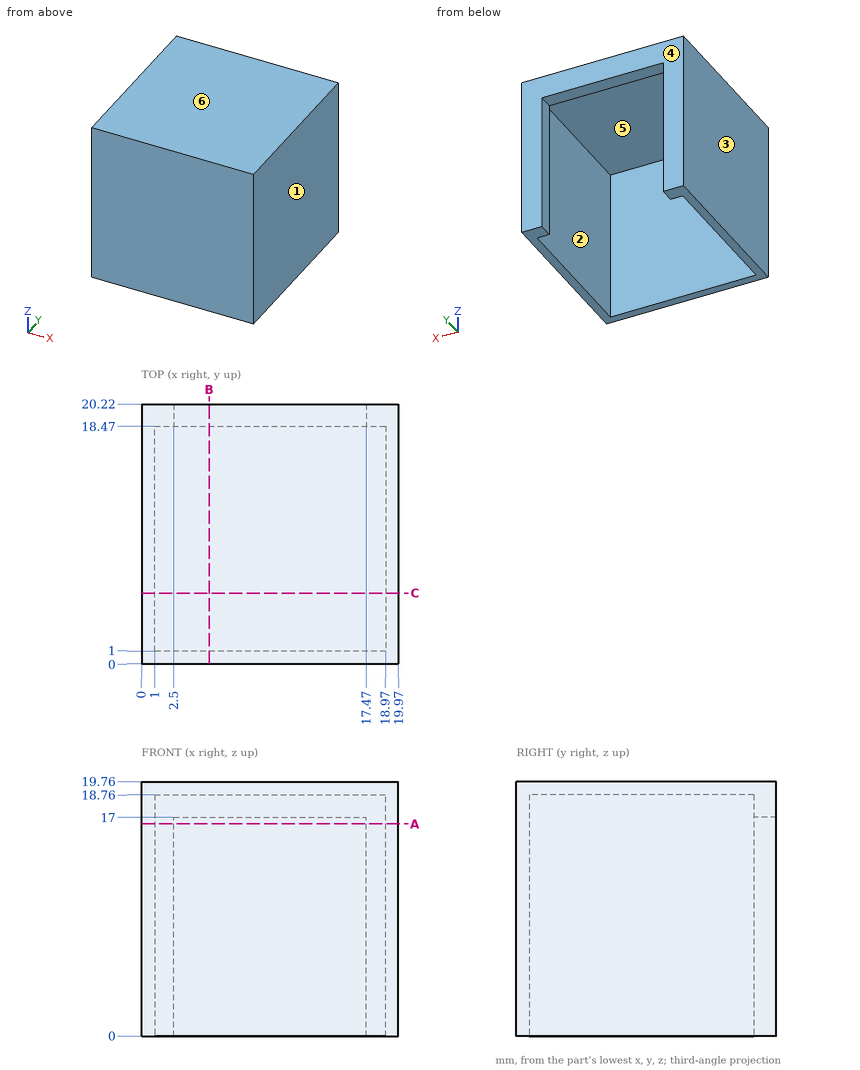
Geometry: see drawing. Coordinates: mm, zero at the bounding-box minimum. A direction names the side the tool comes from. Give positions to 0.01 mm unless a question says otherwise; leave off trailing zeros. Loops run counter-clockwise (first coordinate to the right, second up) from the corner with the lowest first, then second, coordinate; pieces in that order, holes last. Notation, with made-up numbers: (42.5, -31) - (84.5, -31) arc R18 cw to (84.5, -20) - close; hole circle Ø9 at (0.25, 77.25). An arc over 180 degrees is marked (long way). Answer as CSV lines item,"result". Start each with the question number.
1. Draft query along X for the marked faces 1, 2, 3 and 4. Return one class per face: released by +X, released by -X, zero draft, split by the parting line, or undercut.
2. Ray query, L1, parallel to X at y = 18, z = 13.5; L2, parallel to Y at x = 2, z = 13.25; L3, parallel to Z at x = 5.5, y = 5.5. Return the intervals inside material, ascending.
3. Section B-B, the plane x = 5.25. Return loops of the section in (y, z).
4. Section C-C, the plane y = 5.5. Return loops of the section in (x, z).
5. Reachability of the marked faces 5 and 6 from +Z, -Z, +X, -X, +Y, -Y: full face, straight path, thin tool, end or side. Return the list, or none.
6. Pin query (flat end, axial travel): P1, Ø6, axis at y = 8.5, z = 15, coming from the -X side; P2, Ø8.5, axis at x = 9, y = 12, coming from the -Z side; P3, Ø0.5, axis at x = 11.5, y = 19, coming from the -Z side. Return the tip coordinate at first contact, or that it passes through.
7. Section A-A, the plane z = 16.5. Return loops of the section in (x, y).
Answers:
1,face 1,"released by +X"
1,face 2,"undercut"
1,face 3,"released by -X"
1,face 4,"zero draft"
2,L1,"x = 0 to 1, 18.97 to 19.97"
2,L2,"y = 0 to 1, 18.47 to 20.22"
2,L3,"z = 18.76 to 19.76"
3,outline,"(0, 0) - (1, 0) - (1, 18.76) - (18.47, 18.76) - (18.47, 17) - (20.22, 17) - (20.22, 19.76) - (0, 19.76) - close"
4,outline,"(0, 0) - (1, 0) - (1, 18.76) - (18.97, 18.76) - (18.97, 0) - (19.97, 0) - (19.97, 19.76) - (0, 19.76) - close"
5,face 5,"-Z"
5,face 6,"+Z, +X, -X, +Y, -Y"
6,P1,"stops at x = 0"
6,P2,"stops at z = 18.76"
6,P3,"stops at z = 17"
7,outline,"(0, 0) - (19.97, 0) - (19.97, 20.22) - (17.47, 20.22) - (17.47, 18.47) - (18.97, 18.47) - (18.97, 1) - (1, 1) - (1, 18.47) - (2.5, 18.47) - (2.5, 20.22) - (0, 20.22) - close"
